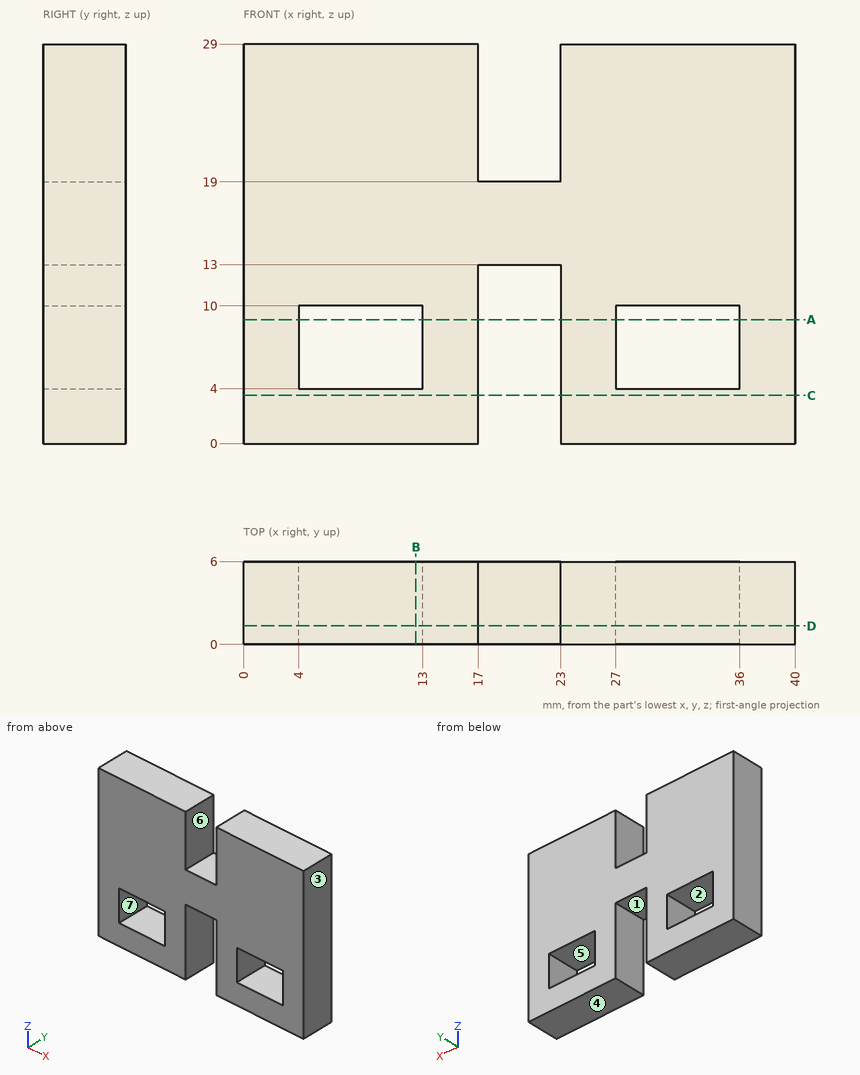
Answer from the drawing. Dimensions are ordinates in mm from the lowest x, y and z of the part. A direction names the side the tool comes from. Coordinates: 2 decimals unless noted, no trailing zeros. Write each loop counter-clockwise with the first axis right and the second up, starting at its lowest first coordinate (ties: lowest second). Pieces come first, ordered by that corner, then holes. Notation, with made-up numbers: (-34.5, 79) - (16.5, 79) arc R23 ccw to (16.5, 100) - close; hole circle Ø9 at (1, 88.5). An arc over 180 degrees is marked (long way). One line per question, with ' | ' between items.
Q1. Determine the mould class of the marked faces 4, 5, 6 and 7 for opening direction Z: +Z half, -Z half, draft (parallel to the pull), parting line (faces both ways), or undercut.
Result set:
face 4: -Z half | face 5: undercut | face 6: draft | face 7: undercut
Q2. Consider L1, parallel to X at y = 5.05, z = 4.5; L2, parallel to Z at x = 6.5, y = 1.4; L3, parallel to X at y = 0.9, z = 2. Determine where each line is inside the solid, lowest interval first. Write a range as [from, to].
Result set:
L1: [0, 4], [13, 17], [23, 27], [36, 40] | L2: [0, 4], [10, 29] | L3: [0, 17], [23, 40]
Q3. Find section B-B, the plane x = 12.5. Write down the section's boundary in (y, z).
Result set:
outline: (0, 0) - (6, 0) - (6, 4) - (0, 4) - close; (0, 10) - (6, 10) - (6, 29) - (0, 29) - close
Q4. Find section C-C, the plane z = 3.5. Write down the section's boundary in (x, y).
Result set:
outline: (0, 0) - (17, 0) - (17, 6) - (0, 6) - close; (23, 0) - (40, 0) - (40, 6) - (23, 6) - close
Q5. Find section A-A, the plane z = 9. Write down the section's boundary in (x, y).
Result set:
outline: (0, 0) - (4, 0) - (4, 6) - (0, 6) - close; (13, 0) - (17, 0) - (17, 6) - (13, 6) - close; (23, 0) - (27, 0) - (27, 6) - (23, 6) - close; (36, 0) - (40, 0) - (40, 6) - (36, 6) - close
Q6. This flat-tipped pin is pushed along its axis until it touches: P1, Ø1.8, axis at y = 3, z = 8.5, coming from the -X side. Where does it stop, or does it pass through?
Result set:
P1: x = 0
Q7. For the marked faces 1, 2 and 3, determine the directions among +Z, -Z, +X, -X, +Y, -Y from which every point of the face is accessible in a straight line to the end or side of a thin tool.
Result set:
face 1: -Z, +Y, -Y | face 2: +Y, -Y | face 3: +Z, -Z, +X, +Y, -Y
Q8. Find section D-D, the plane y = 1.35. Write down the section's boundary in (x, z).
Result set:
outline: (0, 0) - (17, 0) - (17, 13) - (23, 13) - (23, 0) - (40, 0) - (40, 29) - (23, 29) - (23, 19) - (17, 19) - (17, 29) - (0, 29) - close; hole (4, 4) - (13, 4) - (13, 10) - (4, 10) - close; hole (27, 4) - (36, 4) - (36, 10) - (27, 10) - close
